Input: part model. Units: mm. Frame: model coordinates. A direction names the side the tool comes from. Give positions to 0.01 mm unless a question says otherwise; leave off trailing zeros. Answer in a Markdown table with one row per item. Add a question column.
from build123d import *

# Parameters (mm, degrees)
SKETCH1_R           = 1.5
SKETCH1_W           = 10
SKETCH1_H           = 3
SKETCH1_H_2         = 20
BOSS_EXTRUDE1_DEPTH = 10


with BuildPart() as part:
    # Sketch1 → Boss-Extrude1 (new body)
    with BuildSketch(Plane.XY):
        Polygon((-125, -75), (-75, -75), (-75, -72.5), (-65, -72.5), (-65, -75), (-25, -75), (-15, -75), (125, -75), (125, 75), (-15, 75), (-25, 75), (-65, 75), (-65, 72.5), (-75, 72.5), (-75, 75), (-125, 75), align=None)
        with Locations((75.5, 15)):
            Circle(SKETCH1_R, mode=Mode.SUBTRACT)
        with Locations((75.5, -15)):
            Circle(SKETCH1_R, mode=Mode.SUBTRACT)
        with Locations((-117.5, -15)):
            Circle(SKETCH1_R, mode=Mode.SUBTRACT)
        with Locations((-117.5, -45)):
            Circle(SKETCH1_R, mode=Mode.SUBTRACT)
        with Locations((35.010304949, -67.5)):
            Circle(SKETCH1_R, mode=Mode.SUBTRACT)
        with Locations((65.010304949, -67.5)):
            Circle(SKETCH1_R, mode=Mode.SUBTRACT)
        with Locations((35.010304949, 67.5)):
            Circle(SKETCH1_R, mode=Mode.SUBTRACT)
        with Locations((65.010304949, 67.5)):
            Circle(SKETCH1_R, mode=Mode.SUBTRACT)
        with Locations((-117.5, 25.573512729)):
            Circle(SKETCH1_R, mode=Mode.SUBTRACT)
        with Locations((-117.5, 10.573512729)):
            Circle(SKETCH1_R, mode=Mode.SUBTRACT)
        with Locations((-5.559425317, -18.495275092)):
            Circle(SKETCH1_R, mode=Mode.SUBTRACT)
        with Locations((-80.459425317, -18.495275092)):
            Circle(SKETCH1_R, mode=Mode.SUBTRACT)
        with Locations((-86.859425317, 29.304724908)):
            Circle(SKETCH1_R, mode=Mode.SUBTRACT)
        with Locations((-4.259425317, 29.304724908)):
            Circle(SKETCH1_R, mode=Mode.SUBTRACT)
        with Locations((-56.359425317, 24.604724908)):
            Circle(SKETCH1_R, mode=Mode.SUBTRACT)
        with Locations((-56.359425317, -3.295275092)):
            Circle(SKETCH1_R, mode=Mode.SUBTRACT)
        with Locations((92, 15)):
            Circle(SKETCH1_R, mode=Mode.SUBTRACT)
        with Locations((116, 15)):
            Circle(SKETCH1_R, mode=Mode.SUBTRACT)
        with Locations((116, -15)):
            Circle(SKETCH1_R, mode=Mode.SUBTRACT)
        with Locations((92, -15)):
            Circle(SKETCH1_R, mode=Mode.SUBTRACT)
        with Locations((-117.5, 67.5)):
            Circle(SKETCH1_R, mode=Mode.SUBTRACT)
        with Locations((117.5, 68.5)):
            Circle(SKETCH1_R, mode=Mode.SUBTRACT)
        with Locations((117.5, -67.5)):
            Circle(SKETCH1_R, mode=Mode.SUBTRACT)
        with Locations((-117.5, -67.5)):
            Circle(SKETCH1_R, mode=Mode.SUBTRACT)
        with Locations((-70, -53.5)):
            Rectangle(SKETCH1_W, SKETCH1_H, mode=Mode.SUBTRACT)
        with Locations((-70, 53.5)):
            Rectangle(SKETCH1_W, SKETCH1_H, mode=Mode.SUBTRACT)
        with Locations((-50, -55)):
            Rectangle(SKETCH1_W, SKETCH1_H_2, mode=Mode.SUBTRACT)
        with Locations((-50, 55)):
            Rectangle(SKETCH1_W, SKETCH1_H_2, mode=Mode.SUBTRACT)
    extrude(amount=BOSS_EXTRUDE1_DEPTH)


solid = part.part
Q1. Access query for faces 3 (the flat face through (-55, 55, 5)), 4 (the flat face through (29, -75, 5)), 5 (the flat face through (-70, 72.5, 5)), 6 (the flat face through (-70, -72.5, 5)). Directions: +Z, -Z, +X, -X, +Y, -Y. A direction counts if a zero-diameter tool reaches every point of the face in a straight line with its end or side. Return the directions, or none.
Q2. Contact query for flat-ended pins moving along their axis: P1, Ø4, axis at x = -80.46, y = -18.5, coming from the -Z side; P2, Ø1.8, axis at x = 75.5, y = 15, coming from the -Z side. Output: stop coordinate, or through.
Q3. Pull-direction query (X, two-part tool) for faces 1 (the flat face through (-70, 55, 5)), 2 (the flat face through (-100, 75, 5)); classes: +X half, -X half, draft (parallel to the pull), parting line (faces both ways), or undercut.
Q4. Line query: probe 1 along Y at (x, z) = (65, 3.5); probe 2 along Y at (x, z) = (-66, 7); probe 3 along X at (y, z) = (-67.5, 9.5). Output: solid intervals per line, ascending.
Q5. Section A-A, the plane z = 7. State how many separate pieces and enclosed holes the cut face has, then the cut area to 3 significant figures.
Computed:
| question | item | result |
|---|---|---|
| 1 | face 3 | +Z, -Z |
| 1 | face 4 | +Z, -Z, +X, -X, -Y |
| 1 | face 5 | +Z, -Z, +Y |
| 1 | face 6 | +Z, -Z, -Y |
| 2 | P1 | stops at z = 0 |
| 2 | P2 | passes through |
| 3 | face 1 | undercut |
| 3 | face 2 | draft |
| 4 | probe 1 | y = -75 to -69, -66 to 66, 69 to 75 |
| 4 | probe 2 | y = -72.5 to -55, -52 to 52, 55 to 72.5 |
| 4 | probe 3 | x = -125 to -119, -116 to 33.51, 36.51 to 63.51, 66.51 to 116, 119 to 125 |
| 5 | separate pieces | 1 |
| 5 | enclosed holes | 28 |
| 5 | area | 36,800 mm^2 |
